Could you check a few things on this drawing? It's one solid part, dimensions in mm from its lowest x, y, z. Coordinates: 2 decimals unless noted, no trailing zeros. Order: outer loops, then holes, each group sorted by start corner. A loop starts at its lowest first (then second) coordinate and runs counter-clockwise, first axis right, second up. Notation, with made-up numbers: M 81,-21.75 L 90,-21.75 A10 ccw 90,-12.75 Z; hole C -18,0 d11. An arc over 180 degrees is marked long. Answer as CSV lines item,"result". Start each with the question number.
1. If we section it at C-C (y = 29.5): List the corners of the cut face in (x, z) for me.
2. If we section it at A-A (x = 33): List the corners of the cut face in (y, z) for me, plus the area to 3 significant figures.
3. I need wall thicknesses on line 1 along X through (y, z) = (4, 0.5); line 2 along Y through (x, z) = (34, 0.4); line 3 along X through (y, z) = (34.5, 2). Which ranges of each line are inside material? Lowest first, please. Write a range as from..to.
4. Will these pins go through, and if not, where does the flat tip stop? pin 1 (1.5 mm diameter, centred on y = 31.5, z = 2, fed in from -X); pin 2 (0.9 mm diameter, centred on y = 5, z = 2, fed in from +X); pin 3 (1.5 mm diameter, centred on x = 2, z = 1, fed in from +Y).
5. If we section it at B-B (z = 1.05): List the corners of the cut face in (x, y) for me, plus the area to 3 significant figures.
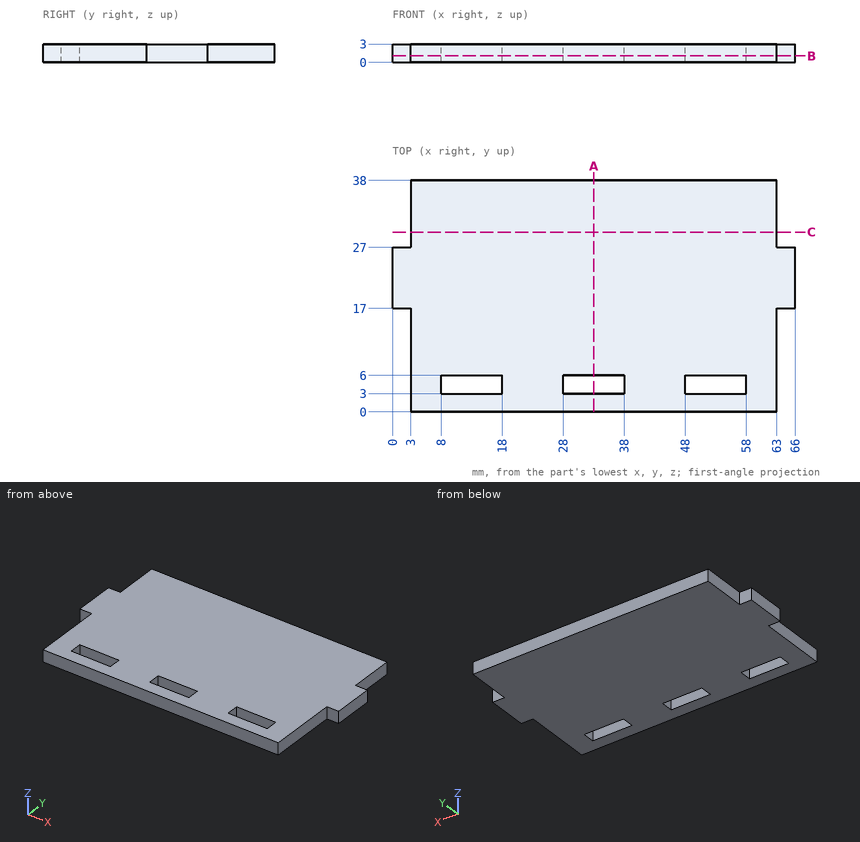
Solved:
1,outline,"M 3,0 L 63,0 L 63,3 L 3,3 Z"
2,outline,"M 0,0 L 3,0 L 3,3 L 0,3 Z; M 6,0 L 38,0 L 38,3 L 6,3 Z"
2,area,"105 mm²"
3,line 1,"3..8, 18..28, 38..48, 58..63"
3,line 2,"0..3, 6..38"
3,line 3,"3..63"
4,pin 1,"x = 3"
4,pin 2,"x = 63"
4,pin 3,"y = 27"
5,outline,"M 0,17 L 3,17 L 3,0 L 63,0 L 63,17 L 66,17 L 66,27 L 63,27 L 63,38 L 3,38 L 3,27 L 0,27 Z; hole M 8,3 L 18,3 L 18,6 L 8,6 Z; hole M 28,3 L 38,3 L 38,6 L 28,6 Z; hole M 48,3 L 58,3 L 58,6 L 48,6 Z"
5,area,"2,250 mm²"
